Build history of the part. All positions in model axes, mm. Give positions to 0.01 mm unless a question says otherwise; leave off trailing zeros. Order: outer loops, then holes, each group sorted by start corner. A loop starts at its lowest first (then second) coordinate and runs counter-clockwise, first axis right, second up. Notation, with made-up numbers: (49.5, 79.5) -> (55.5, 79.5) arc R20 cw to (55.5, 86.5) -> close; hole circle Ø11 at (-0.5, 71.25). An arc over 180 degrees is marked (long way). One line per item, written item: value. Start each with the question number.
(1) Saw through at A-A on z = 0. Give the cut face in (x, y), plus the area to 3 significant figures.
(2) Probe line 1 (X direction, y = 10.85, z = 14); line 2 (Z direction, x = 35, y = 11.3); line 3 (X direction, y = 10.85, z = -38). List the from-to ranges inside material, lowest first.
(3) Saw through at C-C on y = 11.25. Give the cut face in (x, z), plus the area to 3 significant figures.
(4) Saw through at B-B on x = 0. Give the cut face in (y, z), plus the area to 3 significant figures.
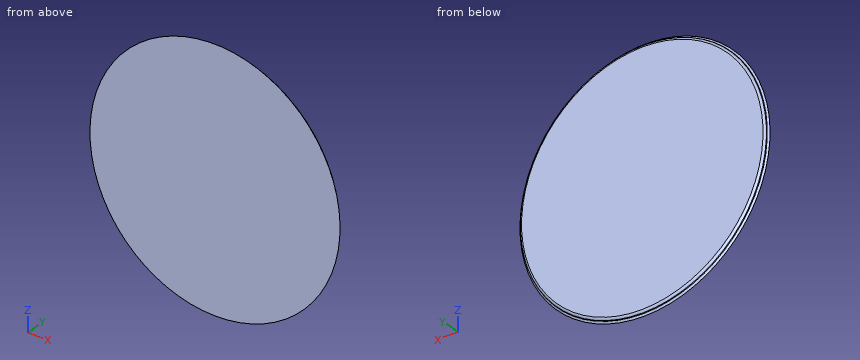
```python
from build123d import *

# Parameters (mm, degrees)
SKIZZE1_R                       = 75
AUFSATZ_LINEAR_AUSTRAGEN1_DEPTH = 10
SKIZZE8_R                       = 75
SCHNITT_LINEAR_AUSTRAGEN1_DEPTH = 10


with BuildPart() as part:
    # Skizze1 → Aufsatz-Linear austragen1 (new body)
    with BuildSketch(Plane(origin=(0, 0, 0), x_dir=(1, 0, 0), z_dir=(0, 1, 0))):
        with Locations(Location((0, 0, 0), (0, 0, 270))):  # turned: the seam where the file's is
            Circle(SKIZZE1_R)
    extrude(amount=AUFSATZ_LINEAR_AUSTRAGEN1_DEPTH)

    # Skizze7 → Rotation1 (revolve)
    with BuildSketch(Plane.XY, mode=Mode.PRIVATE) as rotation1_sk:
        with BuildLine():
            Line((-51.748245903, 10.526383885), (-51.633363701, 10.842020143))
            ThreePointArc((-51.633363701, 10.842020143), (-51.267247516, 11.319152044), (-50.69367108, 11.5))
            Line((-50.69367108, 11.5), (0, 11.5))
            Line((0, 11.5), (0, 10))
            Line((0, 10), (-52.5, 10))
            ThreePointArc((-52.5, 10), (-52.041138851, 10.144678365), (-51.748245903, 10.526383885))
        make_face()
    revolve(rotation1_sk.sketch.rotate(Axis((0, 0, 0), (0, 1, 0)), 270), axis=Axis((0, 0, 0), (0, 1, 0)))  # turned: the seam where the file's is

    # Skizze8 → Schnitt-Linear austragen1 (cut)
    with BuildSketch(Plane.XZ):
        Circle(SKIZZE8_R)
    extrude(amount=-SCHNITT_LINEAR_AUSTRAGEN1_DEPTH, mode=Mode.SUBTRACT)


solid = part.part
```
Results below:
1. outline: (-52.5, 10) -> (52.5, 10) arc R0.8 cw to (51.75, 10.53) -> (51.63, 10.84) arc R1 ccw to (50.69, 11.5) -> (-50.69, 11.5) arc R1 ccw to (-51.63, 10.84) -> (-51.75, 10.53) arc R0.8 cw to start
1. area: 155 mm²
2. line 1: x = -49.7 to 49.7
2. line 2: z = -37.5 to 37.5
2. line 3: x = -34.95 to 34.95
3. outline: circle Ø102.71 at (0, 0)
3. area: 8,290 mm²
4. outline: (10, -52.5) arc R0.8 cw to (10.53, -51.75) -> (10.84, -51.63) arc R1 ccw to (11.5, -50.69) -> (11.5, 50.69) arc R1 ccw to (10.84, 51.63) -> (10.53, 51.75) arc R0.8 cw to (10, 52.5) -> close
4. area: 155 mm²
